Part print with two shaded views. Sizes in mm from the minimum x, y, z corner. Round coordinates to 2 decimals unless told otherwise and drop trailing zeros. Order: outer loops, then holes, each group sorted by start corner. A loop starts at its lowest first (then second) coordinate and runs counter-clockwise, first axis right, second up. Notation, with made-up numbers: M 6.25,33.25 L 46.25,33.25 A32 cw 46.25,69.25 Z; hole C 69,52.5 d9. An arc over 180 degrees is marked long. Return JSON: item names as keys, results as strings. Group by question number.
Item 1: Slice it at A-A on y = 25. Write the cut outline in (x, z).
Item 2: Slice it at D-D on y = 16. Write the cut outline in (x, z), then the cut area to 3 significant figures.
Item 3: Pin check, flat tips, straight feed: pin 1 Ø5 at (y, z) = (44.5, 10.5) entering from +X; pin 2 Ø1 at (y, z) = (25, 37) entering from -X; pin 3 Ø6 at (y, z) = (8, 35.5) entering from +X. Stop position of each tip, or through.
Item 4: Pull direction Z, two halves, no side cores. Call the marked faces 1, 2, 3 and 4: pulls with the +Z half, pulls with the -Z half, needs draft (parallel to the pull), parting line crosses it, or undercut.
Item 5: Probe line 1 along Y through (x, z) = (25, 14); line 2 along Z through (x, y) = (44.5, 14); line 3 along Y through (x, z) = (33, 39). List the from-to ranges inside material, lowest first.
Item 6: Slice it at C-C on z = 7.5. Write the cut outline in (x, y).
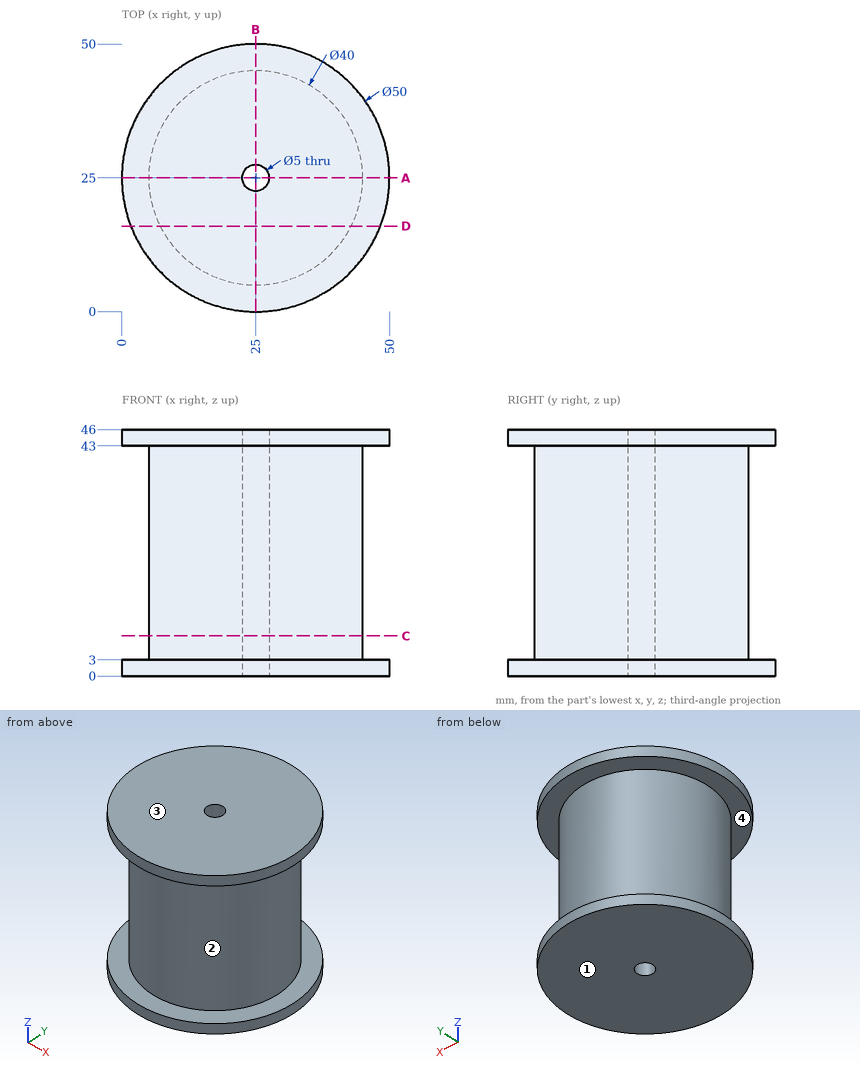
Output values:
{
 "1": {"outline": "M 0,0 L 22.5,0 L 22.5,46 L 0,46 L 0,43 L 5,43 L 5,3 L 0,3 Z; M 27.5,0 L 50,0 L 50,3 L 45,3 L 45,43 L 50,43 L 50,46 L 27.5,46 Z"},
 "2": {"outline": "M 1.68,0 L 48.32,0 L 48.32,3 L 42.86,3 L 42.86,43 L 48.32,43 L 48.32,46 L 1.68,46 L 1.68,43 L 7.14,43 L 7.14,3 L 1.68,3 Z", "area": "1,710 mm²"},
 "3": {"pin 1": "x = 35.54", "pin 2": "x = 5", "pin 3": "x = 39.28"},
 "4": {"face 1": "pulls with the -Z half", "face 2": "undercut", "face 3": "pulls with the +Z half", "face 4": "undercut"},
 "5": {"line 1": "5 to 22.5, 27.5 to 45", "line 2": "0 to 3, 43 to 46", "line 3": "6.67 to 43.33"},
 "6": {"outline": "C 25,25 d40; hole C 25,25 d5"}
}
